from build123d import *

# Parameters (mm, degrees)
SKETCH011_W     = 18.8
SKETCH011_H     = 47
PAD007_DEPTH    = 97.8
SKETCH025_R     = 2
POCKET007_DEPTH = 18.8
SKETCH026_W     = 47
SKETCH026_H     = 42.3
POCKET008_DEPTH = 10.8
SKETCH027_R     = 11
POCKET009_DEPTH = 2.5
SKETCH028_R     = 3.5
POCKET010_DEPTH = 18.801
SKETCH030_W     = 47
SKETCH030_H     = 14.1
POCKET011_DEPTH = 2
SKETCH056_R     = 8
POCKET023_DEPTH = 18.801
SKETCH057_R     = 11
POCKET024_DEPTH = 7
FILLET002_R     = 23.49
SKETCH074_R     = 1.5
POCKET029_DEPTH = 18.801
CHAMFER003_SIZE = 2.5


with BuildPart() as part:
    # Sketch011 (on DatumPlane) → Pad007 (new body)
    with BuildSketch(Plane.XY):
        with Locations((50.4, 0)):
            Rectangle(SKETCH011_W, SKETCH011_H)
    extrude(amount=PAD007_DEPTH)

    # Sketch025 (on Face4 of Pad007) → Pocket007 (cut)
    with BuildSketch(Plane.YZ.offset(59.8)):
        with Locations((-15.5, 55.45)):
            Circle(SKETCH025_R)
        with Locations((15.5, 55.45)):
            Circle(SKETCH025_R)
        with Locations((-15.5, 24.45)):
            Circle(SKETCH025_R)
        with Locations((15.5, 24.45)):
            Circle(SKETCH025_R)
    extrude(amount=-POCKET007_DEPTH, mode=Mode.SUBTRACT)

    # Sketch026 (on Face2 of Pad007) → Pocket008 (cut)
    with BuildSketch(Plane(origin=(41, 0, 0), x_dir=(0, -1, 0), z_dir=(-1, 0, 0))):
        with Locations((0, 39.95)):
            Rectangle(SKETCH026_W, SKETCH026_H)
    extrude(amount=-POCKET008_DEPTH, mode=Mode.SUBTRACT)

    # Sketch027 (on Face5 of Pocket008) → Pocket009 (cut)
    with BuildSketch(Plane(origin=(51.8, 0, 0), x_dir=(0, -1, 0), z_dir=(-1, 0, 0))):
        with Locations((0, 39.95)):
            Circle(SKETCH027_R)
    extrude(amount=-POCKET009_DEPTH, mode=Mode.SUBTRACT)

    # Sketch028 (on Face7 of Pocket009) → Pocket010 (cut, through all)
    with BuildSketch(Plane(origin=(41, 0, 0), x_dir=(0, -1, 0), z_dir=(-1, 0, 0))):
        with Locations((0, 39.95)):
            Circle(SKETCH028_R)
    extrude(amount=-POCKET010_DEPTH, mode=Mode.SUBTRACT)

    # Sketch030 (on Face3 of Pocket007) → Pocket011 (cut)
    with BuildSketch(Plane(origin=(41, 0, 0), x_dir=(0, -1, 0), z_dir=(-1, 0, 0))):
        with Locations((0, 7.05)):
            Rectangle(SKETCH030_W, SKETCH030_H)
    extrude(amount=-POCKET011_DEPTH, mode=Mode.SUBTRACT)

    # Sketch056 (on Face11 of Pocket011) → Pocket023 (cut, through all)
    with BuildSketch(Plane.YZ.offset(59.8)):
        with Locations((0, 75)):
            Circle(SKETCH056_R)
    extrude(amount=-POCKET023_DEPTH, mode=Mode.SUBTRACT)

    # Sketch057 (on Face11 of Pocket023) → Pocket024 (cut)
    with BuildSketch(Plane.YZ.offset(59.8)):
        with Locations((0, 75)):
            Circle(SKETCH057_R)
    extrude(amount=-POCKET024_DEPTH, mode=Mode.SUBTRACT)

    # Fillet002
    fillet002_edges = [part.edges().sort_by_distance(p)[0] for p in [
        (50.4, 23.5, 97.8),
        (50.4, -23.5, 97.8),
    ]]
    fillet(fillet002_edges, radius=FILLET002_R)

    # Sketch074 (on Face5 of Fillet002) → Pocket029 (cut, through all)
    with BuildSketch(Plane.YZ.offset(59.8)):
        with Locations((-11.75, 9.4)):
            Circle(SKETCH074_R)
        with Locations((11.75, 9.4)):
            Circle(SKETCH074_R)
    extrude(amount=-POCKET029_DEPTH, mode=Mode.SUBTRACT)

    # Chamfer003
    chamfer003_edges = [part.edges().sort_by_distance(p)[0] for p in [
        (59.8, 10.25, 9.4),
        (59.8, -13.25, 9.4),
    ]]
    chamfer(chamfer003_edges, length=CHAMFER003_SIZE)


solid = part.part
CAD build for the part. Positions are in the model's coordinates, mm. A direction names the side the tool comes from. Give positions to 0.01 mm unless a question says otherwise; leave off trailing zeros. Loops run counter-clockwise (first coordinate to the right, second up) from the corner with the lowest first, then second, coordinate; pieces in that order, holes last. Notation, with made-up numbers: M 81.5,43.5 L 90.5,43.5 A4 cw 90.5,48.5 Z; hole C -1.5,-30 d7. An arc over 180 degrees is marked long. Write each question's results on one line, items separated by ' | '.
Q1. Band-saw the part on C-C on z = 39.95. Write the cut outline in (x, y).
Geometry check:
outline: M 51.8,-23.5 L 59.8,-23.5 L 59.8,-3.5 L 54.3,-3.5 L 54.3,-11 L 51.8,-11 Z; M 51.8,11 L 54.3,11 L 54.3,3.5 L 59.8,3.5 L 59.8,23.5 L 51.8,23.5 Z
Q2. Mould opens along Y. For faces 1 (the face through (50.53, 16.8, 90.74)), 2 (the face through (57.42, -12.1, 7.82)), 3 (the face through (51.8, 6, 50)) say: pulls with the +Y half, pulls with the -Y half, needs draft (parallel to the pull), parting line crosses it, or undercut.
Geometry check:
face 1: pulls with the +Y half | face 2: undercut | face 3: needs draft
Q3. Band-saw the part on B-B on z = 9.4. Write the cut outline in (x, y), and give its area (3 significant figures).
Geometry check:
outline: M 43,-23.5 L 59.8,-23.5 L 59.8,-15.75 L 57.3,-13.25 L 43,-13.25 Z; M 43,-10.25 L 57.3,-10.25 L 59.8,-7.75 L 59.8,7.75 L 57.3,10.25 L 43,10.25 Z; M 43,13.25 L 57.3,13.25 L 59.8,15.75 L 59.8,23.5 L 43,23.5 Z | area: 676 mm²
Q4. Band-saw the part on A-A on x = 44.75. Give the number of separate pieces and of enclosed holes in the cut face, and give its area (3 significant figures).
Geometry check:
separate pieces: 2 | enclosed holes: 3 | area: 2,160 mm²
Q5. Which spindle directions (+Z, -Z, +X, -X, +Y, -Y) get a long thin tool onto all of the face, cutting with end or side? Do faces 4 (the face through (56.349, -1.432, 85.906)), 5 (the face through (46, 0, 18.8)), 6 (the face through (42, 0, 14.1)). Say none if no direction does.
Geometry check:
face 4: +X | face 5: -X, +Y, -Y | face 6: -Z, -X, +Y, -Y
Q6. Flat gauge pins, fed straight in: P1, Ø24, axis at y = -1.5, z = 45.5, coming from the -X side; P2, Ø5, axis at y = 11.75, z = 9.4, coming from the -X side; P3, Ø2.5, axis at y = -11.75, z = 9.4, coming from the +X side; P4, Ø1, axis at x = 44, z = 81, coming from the -Y side. Where does each tip first touch, or does it go through?
Geometry check:
P1: stops at x = 51.8 | P2: stops at x = 43 | P3: passes through | P4: stops at y = -22.67
Q7. Probe probe 1 along Y at (x, z) = (52.5, 55.5); probe 2 along Z at (x, y) = (58, 0); probe 3 along Y at (x, z) = (52, 25). List the from-to ranges inside material, lowest first.
Geometry check:
probe 1: y = -23.5 to -17.5, -13.5 to 13.5, 17.5 to 23.5 | probe 2: z = 0 to 36.45, 43.45 to 64, 86 to 97.8 | probe 3: y = -23.5 to -17.42, -13.58 to 13.58, 17.42 to 23.5
